Check sheet for the modelled part. Datum: model origin and axes. Units: mm. A direction names the side the tool comes from. Round coordinates to 2 decimals unless told otherwise and drop trailing zeros. Order: outer loops, then holes, each group sorted by start corner. A loop starts at its lowest first (then second) coordinate and runs counter-clockwise, first axis right, second up. Notation, with made-up numbers: (55.5, -21) -> (98.5, -21) arc R18 ccw to (98.5, -16) -> close; hole circle Ø1 at (-25.75, -19). An arc over 180 degrees is marked (long way). Answer in a Markdown table with one row per item.
```python
from build123d import *

# Parameters (mm, degrees)
SKETCH_324_R             = 1.5
EXTRUDE_1_DEPTH          = 3
SKETCH_2_R               = 1.5
CUT_EXTRUDE_1_DEPTH      = 111.5
CUT_EXTRUDE_1_DEPTH_BACK = 41.5
CUT_EXTRUDE_2_DEPTH      = 1.5
SKETCH_6_R               = 1.5
CUT_EXTRUDE_3_DEPTH      = 2.5
SKETCH_8_R               = 3.075
EXTRUDE_3_DEPTH          = 16.35
MIRROR_8_COPY_1_SKETCH_R = 3.075
MIRROR_8_COPY_1_DEPTH    = 16.35
MIRROR_8_COPY_2_SKETCH_R = 3.075
MIRROR_8_COPY_2_DEPTH    = 16.35
SKETCH_11_R              = 1.5
CUT_EXTRUDE_4_DEPTH      = 41.5


with BuildPart() as part:
    # Sketch 324 → 填料-伸長1 (new body)
    with BuildSketch(Plane.XY):
        with BuildLine():
            ThreePointArc((100.510480498, -70.70616545), (102.320143894, -72.389238388), (104.714843536, -73))
            Line((104.714843536, -73), (126.986921935, -73))
            Line((126.986921935, -73), (126.986921935, -80))
            Line((126.986921935, -80), (98.725740556, -80))
            ThreePointArc((98.725740556, -80), (93.936341272, -78.778476776), (90.317014479, -75.4123309))
            Line((90.317014479, -75.4123309), (54.385110012, -19.5876691))
            ThreePointArc((54.385110012, -19.5876691), (50.76578322, -16.221523224), (45.976383936, -15))
            Line((45.976383936, -15), (2.168890098, -15))
            Line((2.168890098, -15), (0, -15))
            ThreePointArc((0, -15), (-7.5, -7.5), (0, 0))
            Line((0, 0), (49.544156798, 0))
            ThreePointArc((49.544156798, 0), (54.333556082, -1.221523224), (57.952882875, -4.5876691))
            Line((57.952882875, -4.5876691), (100.510480498, -70.70616545))
        make_face()
        with Locations((0, -7.5)):
            Circle(SKETCH_324_R, mode=Mode.SUBTRACT)
    extrude_1 = extrude(amount=EXTRUDE_1_DEPTH)

    # 草圖2 → 除料-伸長1 (cut, two sides)
    with BuildSketch(Plane.XY.offset(3)) as cut_extrude_1_sk:
        with Locations((122.206921935, -76.5)):
            Circle(SKETCH_2_R)
    extrude(amount=CUT_EXTRUDE_1_DEPTH, mode=Mode.SUBTRACT)
    extrude(cut_extrude_1_sk.sketch, amount=-CUT_EXTRUDE_1_DEPTH_BACK, mode=Mode.SUBTRACT)

    # 草圖5 → 除料-伸長2 (cut)
    with BuildSketch(Plane.XY.offset(3)):
        with BuildLine():
            Line((1.802775638, -4.5), (15.929780582, -4.5))
            Line((15.929780582, -4.5), (15.929780582, -10.5))
            Line((15.929780582, -10.5), (1.802775638, -10.5))
            ThreePointArc((1.802775638, -10.5), (-3.5, -7.5), (1.802775638, -4.5))
        make_face()
    extrude(amount=-CUT_EXTRUDE_2_DEPTH, mode=Mode.SUBTRACT)

    # 草圖6 → 除料-伸長3 (cut, through all)
    with BuildSketch(Plane.XY.offset(1.5)):
        with Locations((10.5, -7.5)):
            Circle(SKETCH_6_R)
    extrude(amount=-CUT_EXTRUDE_3_DEPTH, mode=Mode.SUBTRACT)

    # 草圖8 → 填料-伸長3 (add)
    with BuildSketch(Plane.XY.offset(3)):
        with Locations((51.04897254, -7.515441374)):
            Circle(SKETCH_8_R)
    extrude_3 = extrude(amount=EXTRUDE_3_DEPTH)

    # 鏡射7: 填料-伸長3 across plane
    add(extrude_3.mirror(Plane.XY.offset(19.35)))

    # 鏡射8: 填料-伸長1 across plane
    add(extrude_1.mirror(Plane.XY.offset(19.35)))

    # 鏡射8 copy 1 sketch → 鏡射8 copy 1 (add)
    with BuildSketch(Plane.XY.offset(3)):
        with Locations((51.04897254, -7.515441374)):
            Circle(MIRROR_8_COPY_1_SKETCH_R)
    extrude(amount=MIRROR_8_COPY_1_DEPTH)

    # 鏡射8 copy 2 sketch → 鏡射8 copy 2 (add)
    with BuildSketch(Plane(origin=(0, 0, 35.7), x_dir=(1, 0, 0), z_dir=(0, 0, -1))):
        with Locations((51.04897254, 7.515441374)):
            Circle(MIRROR_8_COPY_2_SKETCH_R)
    extrude(amount=MIRROR_8_COPY_2_DEPTH)

    # 草圖11 → 除料-伸長4 (cut)
    with BuildSketch(Plane(origin=(0, 0, 35.7), x_dir=(-1, 0, 0), z_dir=(0, 0, -1))):
        with Locations((-122.206921935, -76.5)):
            Circle(SKETCH_11_R)
    extrude(amount=-CUT_EXTRUDE_4_DEPTH, mode=Mode.SUBTRACT)


solid = part.part
```
(1) Tool access check on faces 5 (the cylindrical face through (53.98, -6.59, 19.12)), 6 (the flat face through (24, 0, 37)), 7 (the flat face through (23, -15, 37)). Record the directions out of +Z, -Z, +X, -X, +Y, -Y that give a thin tool (end or side, any length) a straight path to the whole face; none if there is none.
Solutions:
| item | result |
|---|---|
| face 5 | none |
| face 6 | +Z, -Z, +X, -X, +Y |
| face 7 | +Z, -Z, -X, -Y |
(2) Section check A-A on x = 10.5. Record the boundary of the cut face in (y, z).
Solutions:
| item | result |
|---|---|
| outline | (-15, 0) -> (-9, 0) -> (-9, 1.5) -> (-10.5, 1.5) -> (-10.5, 3) -> (-15, 3) -> close; (-15, 35.7) -> (0, 35.7) -> (0, 38.7) -> (-15, 38.7) -> close; (-6, 0) -> (0, 0) -> (0, 3) -> (-4.5, 3) -> (-4.5, 1.5) -> (-6, 1.5) -> close |
(3) Depth check by flat-ended pin: pin 1 Ø9 at (x, y) = (0, -7.5) entering from -Z; pin 2 Ø3.5 at (x, z) = (25.5, 1) entering from -Y; pin 3 Ø10 at (x, z) = (97, 33) entering from +Y; pin 4 Ø5 at (y, z) = (-11.5, 19) entering from -X. Enter the tip coordinate at first touch or a pass-through.
Solutions:
| item | result |
|---|---|
| pin 1 | z = 0 |
| pin 2 | y = -15 |
| pin 3 | y = -58.71 |
| pin 4 | x = 48.36 |
(4) Draft check along X on faces 1 (the flat face through (116, -73, 37)), 2 (the cylindrical face through (93.998, -78.812, 1.479)), 3 (the flat face through (78.93, -37.18, 37.22)), 4 (the cylindrical face through (-3.5, -7.6, 2.3)). Enter one of: pulls with the +X half, pulls with the -X half, needs draft (parallel to the pull), parting line crosses it, or undercut.
Solutions:
| item | result |
|---|---|
| face 1 | needs draft |
| face 2 | pulls with the -X half |
| face 3 | pulls with the +X half |
| face 4 | undercut |
(5) Scan lines: probe 1 along Y at (x, z) = (10.5, 0.9); probe 2 along Z at (x, y) = (83.5, -57); probe 3 along X at (y, z) = (-7, 1). Record each from-to range of solid material in increasing order. Write a range as from..to.
Solutions:
| item | result |
|---|---|
| probe 1 | -15..-9, -6..0 |
| probe 2 | 0..3, 35.7..38.7 |
| probe 3 | -7.48..-1.41, 1.41..9.09, 11.91..59.51 |
(6) Section check C-C on y = -44. Record the boundary of the cut face in (x, z), plus the area to 3 significant figures.
Solutions:
| item | result |
|---|---|
| outline | (70.1, 0) -> (83.32, 0) -> (83.32, 3) -> (70.1, 3) -> close; (70.1, 35.7) -> (83.32, 35.7) -> (83.32, 38.7) -> (70.1, 38.7) -> close |
| area | 79.3 mm^2 |
(7) Section check B-B on x = 114. Record the boundary of the cut face in (y, z), plus the area to 3 significant figures.
Solutions:
| item | result |
|---|---|
| outline | (-80, 0) -> (-73, 0) -> (-73, 3) -> (-80, 3) -> close; (-80, 35.7) -> (-73, 35.7) -> (-73, 38.7) -> (-80, 38.7) -> close |
| area | 42.0 mm^2 |
(8) Section check D-D on z = 27. Record the boundary of the cut face in (x, y) (3 decimals).
Solutions:
| item | result |
|---|---|
| outline | circle Ø6.15 at (51.049, -7.515) |
